Source: CAD feature listing. Evaluate the final solid. Frame: model axes, mm. Round coordinates to 2 decimals unless told otherwise and drop trailing zeros. Order: outer loops, then holes, each group sorted by start corner. A loop starts at its lowest first (then second) coordinate and runs counter-clockwise, first axis right, second up. Notation, with made-up numbers: (-16, 73.25) - (36, 73.25) arc R10 cw to (36, 78.25) - close; hole circle Ø11 at (-35, 69). An arc over 180 degrees is marked (long way). Put each result on its own line as item: value. Start each with the question number.
1) Line query: probe 1 along X at (y, z) = (1.25, -38); probe 2 along Z at (x, y) = (-85, 3.25); probe 3 along Z at (x, y) = (-31, 2). Output: solid intervals per line, ascending. Write a range as [from, to].
2) Section C-C on y = 3.25. State how many separate pieces and enclosed holes the cut face has, then the cut area to 3 significant figures.
3) Section B-B on x = -69. Output: boundary loops of the cut face in (y, z), then the cut area to 3 significant figures.
4) Section A-A on z = -100. Output: boundary loops of the cut face in (x, y) (3 decimals), then the cut area to 3 significant figures.
5) Contact query for flat-ended pins moving along their axis: P1, Ø3.5, axis at x = -78.69, z = -200, coming from the -Y side; P2, Ø2.5, axis at y = 4, z = 1, coming from the +X side; P3, Ø1.5, axis at y = 0.5, z = -152, coming from the -X side; P4, Ø2, axis at x = -190, y = 4, coming from the -Z side. Output: stop coordinate, or through.
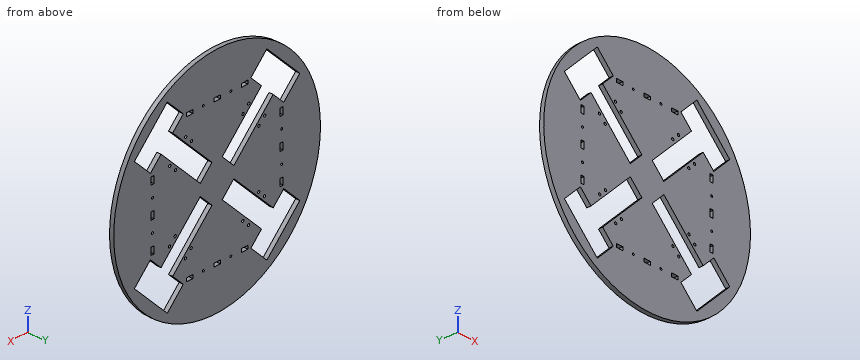
```python
from build123d import *

# Parameters (mm, degrees)
SKETCH1_R           = 160
BOSS_EXTRUDE1_DEPTH = 6
CUT_EXTRUDE1_DEPTH  = 368.744476505
CUT_EXTRUDE2_DEPTH  = 368.744476505
SKETCH7_R           = 1.75
CUT_EXTRUDE3_DEPTH  = 368.744476505
SKETCH9_R           = 1.5
SKETCH9_W           = 4.75
SKETCH9_H           = 10
SKETCH9_W_2         = 10
SKETCH9_H_2         = 4.75
CUT_EXTRUDE4_DEPTH  = 368.744476505


with BuildPart() as part:
    # Sketch1 → Boss-Extrude1 (new body)
    with BuildSketch(Plane(origin=(0, 0, 0), x_dir=(1, 0, 0), z_dir=(0, 1, 0))):
        with Locations(Location((-100, 100, 0), (0, 0, 270))):
            Circle(SKETCH1_R)
    extrude(amount=BOSS_EXTRUDE1_DEPTH)

    # Sketch3 → Cut-Extrude1 (cut, through all)
    with BuildSketch(Plane.XZ):
        Polygon((-22.925360851, -227.986327395), (-47.674098192, -203.237590053), (3.237590053, -152.325901808), (27.986327395, -177.074639149), align=None)
        Polygon((3.237590053, -47.674098192), (27.986327395, -22.925360851), (-22.925360851, 27.986327395), (-47.674098192, 3.237590053), align=None)
        Polygon((-152.325901808, 3.237590053), (-177.074639149, 27.986327395), (-227.986327395, -22.925360851), (-203.237590053, -47.674098192), align=None)
        Polygon((-177.074639149, -227.986327395), (-152.325901808, -203.237590053), (-203.237590053, -152.325901808), (-227.986327395, -177.074639149), align=None)
    extrude(amount=-CUT_EXTRUDE1_DEPTH, mode=Mode.SUBTRACT)

    # Sketch4 → Cut-Extrude2 (cut, through all)
    with BuildSketch(Plane.XZ):
        Polygon((-31.23386553, -186.797357391), (-13.202642609, -168.76613447), (-74.013825791, -107.954951288), (-92.045048712, -125.986174209), align=None)
        Polygon((-125.986174209, -107.954951288), (-186.797357391, -168.76613447), (-168.76613447, -186.797357391), (-107.954951288, -125.986174209), align=None)
        Polygon((-107.954951288, -74.013825791), (-168.76613447, -13.202642609), (-186.797357391, -31.23386553), (-125.986174209, -92.045048712), align=None)
        Polygon((-74.013825791, -92.045048712), (-13.202642609, -31.23386553), (-31.23386553, -13.202642609), (-92.045048712, -74.013825791), align=None)
    extrude(amount=-CUT_EXTRUDE2_DEPTH, mode=Mode.SUBTRACT)

    # Sketch7 → Cut-Extrude3 (cut, through all)
    with BuildSketch(Plane.XZ):
        with Locations(Location((-149.002499936, -26.673026791, 0), (0, 0, 270))):
            Circle(SKETCH7_R)
        with Locations(Location((-148.578235868, -173.751237278, 0), (0, 0, 270))):
            Circle(SKETCH7_R)
        with Locations(Location((-140.163665171, -35.511861556, 0), (0, 0, 270))):
            Circle(SKETCH7_R)
        with Locations(Location((-164.912402513, -60.260598897, 0), (0, 0, 270))):
            Circle(SKETCH7_R)
        with Locations(Location((-173.751237278, -51.421764132, 0), (0, 0, 270))):
            Circle(SKETCH7_R)
        with Locations(Location((-173.326973209, -149.002499936, 0), (0, 0, 270))):
            Circle(SKETCH7_R)
        with Locations(Location((-164.488138444, -140.163665171, 0), (0, 0, 270))):
            Circle(SKETCH7_R)
        with Locations(Location((-139.739401103, -164.912402513, 0), (0, 0, 270))):
            Circle(SKETCH7_R)
        with Locations(Location((-26.673026791, -50.997500064, 0), (0, 0, 270))):
            Circle(SKETCH7_R)
        with Locations(Location((-35.511861556, -59.836334829, 0), (0, 0, 270))):
            Circle(SKETCH7_R)
        with Locations(Location((-60.260598897, -35.087597487, 0), (0, 0, 270))):
            Circle(SKETCH7_R)
        with Locations(Location((-51.421764132, -26.248762722, 0), (0, 0, 270))):
            Circle(SKETCH7_R)
        with Locations(Location((-50.997500064, -173.326973209, 0), (0, 0, 270))):
            Circle(SKETCH7_R)
        with Locations(Location((-59.836334829, -164.488138444, 0), (0, 0, 270))):
            Circle(SKETCH7_R)
        with Locations(Location((-35.087597487, -139.739401103, 0), (0, 0, 270))):
            Circle(SKETCH7_R)
        with Locations(Location((-26.248762722, -148.578235868, 0), (0, 0, 270))):
            Circle(SKETCH7_R)
    extrude(amount=-CUT_EXTRUDE3_DEPTH, mode=Mode.SUBTRACT)

    # Sketch9 → Cut-Extrude4 (cut, through all)
    with BuildSketch(Plane.XZ):
        with Locations(Location((0, -78.6875, 0), (0, 0, 270))):
            Circle(SKETCH9_R)
        with Locations(Location((0, -121.3125, 0), (0, 0, 270))):
            Circle(SKETCH9_R)
        with Locations(Location((-78.6875, -200, 0), (0, 0, 270))):
            Circle(SKETCH9_R)
        with Locations(Location((-121.3125, -200, 0), (0, 0, 270))):
            Circle(SKETCH9_R)
        with Locations(Location((-200, -121.3125, 0), (0, 0, 270))):
            Circle(SKETCH9_R)
        with Locations(Location((-200, -78.6875, 0), (0, 0, 270))):
            Circle(SKETCH9_R)
        with Locations(Location((-121.3125, 0, 0), (0, 0, 270))):
            Circle(SKETCH9_R)
        with Locations(Location((-78.6875, 0, 0), (0, 0, 270))):
            Circle(SKETCH9_R)
        with Locations((0, -142.625)):
            Rectangle(SKETCH9_W, SKETCH9_H)
        with Locations((0, -100)):
            Rectangle(SKETCH9_W, SKETCH9_H)
        with Locations((0, -57.375)):
            Rectangle(SKETCH9_W, SKETCH9_H)
        with Locations((-100, -200)):
            Rectangle(SKETCH9_W_2, SKETCH9_H_2)
        with Locations((-57.375, -200)):
            Rectangle(SKETCH9_W_2, SKETCH9_H_2)
        with Locations((-142.625, -200)):
            Rectangle(SKETCH9_W_2, SKETCH9_H_2)
        with Locations((-200, -100)):
            Rectangle(SKETCH9_W, SKETCH9_H)
        with Locations((-200, -142.625)):
            Rectangle(SKETCH9_W, SKETCH9_H)
        with Locations((-200, -57.375)):
            Rectangle(SKETCH9_W, SKETCH9_H)
        with Locations((-100, 0)):
            Rectangle(SKETCH9_W_2, SKETCH9_H_2)
        with Locations((-142.625, 0)):
            Rectangle(SKETCH9_W_2, SKETCH9_H_2)
        with Locations((-57.375, 0)):
            Rectangle(SKETCH9_W_2, SKETCH9_H_2)
    extrude(amount=-CUT_EXTRUDE4_DEPTH, mode=Mode.SUBTRACT)


solid = part.part
```
Answer sheet:
1. probe 1: [-247.5, -212.91], [-193.56, -180.03], [-143.97, -56.03], [-19.97, -6.44], [12.91, 47.5]
1. probe 2: [-259.3, -133.03], [-118.94, -81.06], [-66.97, 59.3]
1. probe 3: [-244.36, -219.91], [-150.97, -49.03], [19.91, 44.36]
2. separate pieces: 1
2. enclosed holes: 40
2. area: 60,800 mm^2
3. outline: (0, -256.97) - (6, -256.97) - (6, -149.03) - (0, -149.03) - close; (0, -112.97) - (6, -112.97) - (6, -87.03) - (0, -87.03) - close; (0, -50.97) - (6, -50.97) - (6, 56.97) - (0, 56.97) - close
3. area: 1,450 mm^2
4. outline: (-260, 0) - (-202.375, 0) - (-202.375, 6) - (-260, 6) - close; (-197.625, 0) - (-2.375, 0) - (-2.375, 6) - (-197.625, 6) - close; (2.375, 0) - (60, 0) - (60, 6) - (2.375, 6) - close
4. area: 1,860 mm^2
5. P1: y = 0
5. P2: x = 25.1
5. P3: x = -251.57
5. P4: z = -232.96
